Here's how the part is built. I have some questions about the finished solid (model axes, mm). A direction names the side the tool comes from. Round coordinates to 2 decimals unless told otherwise and drop trailing zeros. Write each loop counter-clockwise with the first axis right and the second up, starting at its lowest first coordinate (ties: lowest second). Pieces come first, ordered by that corner, then holes. Notation, with made-up numbers: (24, 25.25) -> (82, 25.25) arc R27 ccw to (82, 48.25) -> close; hole circle Ø2 at (71, 44.5). An arc over 180 degrees is marked (long way). Answer in a Markdown table with one row per item.
from build123d import *

# Parameters (mm, degrees)
SKETCH1_W           = 10
SKETCH1_H           = 14
SKETCH1_R           = 2.1
BOSS_EXTRUDE1_DEPTH = 2
SKETCH2_W           = 1.8
SKETCH2_H           = 13.4
BOSS_EXTRUDE2_DEPTH = 5
SKETCH3_W           = 1.8
SKETCH3_H           = 1.8
CUT_EXTRUDE1_DEPTH  = 9
SKETCH5_W           = 12.2
SKETCH5_H           = 17
BOSS_EXTRUDE4_DEPTH = 2
SKETCH6_W           = 14
SKETCH6_H           = 5
SKETCH6_W_2         = 0.5
CUT_EXTRUDE2_DEPTH  = 14
SKETCH7_W           = 10
SKETCH7_H           = 2
BOSS_EXTRUDE5_DEPTH = 3


with BuildPart() as part:
    # Sketch1 → Boss-Extrude1 (new body)
    with BuildSketch(Plane(origin=(0, 0, 0), x_dir=(1, 0, 0), z_dir=(0, 1, 0))):
        Rectangle(SKETCH1_W, SKETCH1_H)
        Circle(SKETCH1_R, mode=Mode.SUBTRACT)
        Polygon((5, 7), (5, -7), (5, -8.5), (19, -8.5), (19, 8.5), (5, 8.5), align=None)
    extrude(amount=BOSS_EXTRUDE1_DEPTH)

    # Sketch2 → Boss-Extrude2 (add)
    with BuildSketch(Plane(origin=(0, 2, 0), x_dir=(1, 0, 0), z_dir=(0, 1, 0))):
        Polygon((17.2, 6.7), (19, 6.7), (19, 8.5), (5, 8.5), (5, 7), (5, 6.7), align=None)
        with Locations((18.1, 0)):
            Rectangle(SKETCH2_W, SKETCH2_H)
        Polygon((5, -7), (5, -8.5), (19, -8.5), (19, -6.7), (17.2, -6.7), (5, -6.7), align=None)
    extrude(amount=BOSS_EXTRUDE2_DEPTH)

    # Sketch3 → Cut-Extrude1 (cut)
    with BuildSketch(Plane(origin=(0, 7, 0), x_dir=(1, 0, 0), z_dir=(0, 1, 0))):
        Polygon((19, -6.7), (19, 8.5), (17.2, 8.5), (17.2, 6.7), (17.2, -6.7), align=None)
        with Locations((18.1, -7.6)):
            Rectangle(SKETCH3_W, SKETCH3_H)
    extrude(amount=-CUT_EXTRUDE1_DEPTH, mode=Mode.SUBTRACT)

    # Sketch5 → Boss-Extrude4 (add)
    with BuildSketch(Plane(origin=(0, 7, 0), x_dir=(1, 0, 0), z_dir=(0, 1, 0))):
        with Locations((11.1, 0)):
            Rectangle(SKETCH5_W, SKETCH5_H)
    extrude(amount=BOSS_EXTRUDE4_DEPTH)

    # Sketch6 → Cut-Extrude2 (cut)
    with BuildSketch(Plane.ZY.offset(-5)):
        with Locations((0, 4.5)):
            Rectangle(SKETCH6_W, SKETCH6_H)
        with Locations((-7.25, 4.5)):
            Rectangle(SKETCH6_W_2, SKETCH6_H)
        with Locations((7.25, 4.5)):
            Rectangle(SKETCH6_W_2, SKETCH6_H)
    extrude(amount=-CUT_EXTRUDE2_DEPTH, mode=Mode.SUBTRACT)

    # Sketch7 → Boss-Extrude5 (add)
    with BuildSketch(Plane(origin=(0, 0, -7), x_dir=(-1, 0, 0), z_dir=(0, 0, -1))):
        with Locations((0, 1)):
            Rectangle(SKETCH7_W, SKETCH7_H)
    extrude(amount=BOSS_EXTRUDE5_DEPTH)


solid = part.part
1) I want a section at B-B, the plane z = -2.5. List the corners of the cut face in (x, y) for me, and give its area (3 significant figures).
Response:
| item | result |
|---|---|
| outline | (-5, 0) -> (17.2, 0) -> (17.2, 2) -> (-5, 2) -> close; (5, 7) -> (17.2, 7) -> (17.2, 9) -> (5, 9) -> close |
| area | 68.8 mm^2 |
2) I need wall thicknesses on line 1 (X direction, y = 1.3, z = 0); line 2 (Y direction, x = 15.25, z = -2.5); line 3 (Z direction, x = 0, y = 1.2). Which ranges of each line are inside material? Lowest first, please. Write a range as [from, to].
Response:
| item | result |
|---|---|
| line 1 | x = [-5, -2.1], [2.1, 17.2] |
| line 2 | y = [0, 2], [7, 9] |
| line 3 | z = [-10, -2.1], [2.1, 7] |
3) I want a section at A-A, the plane x = 0. List the corners of the cut face in (y, z) for me.
Response:
| item | result |
|---|---|
| outline | (0, -10) -> (2, -10) -> (2, -2.1) -> (0, -2.1) -> close; (0, 2.1) -> (2, 2.1) -> (2, 7) -> (0, 7) -> close |
4) For pin 1 (2.5 mm diameter, centred on x = 13.5, y = 5, fed in from -Z); pin 2 (1.5 mm diameter, centred on x = 0, z = -8, fed in from +Y); pin 3 (4 mm diameter, centred on x = 0, z = 0, fed in from +Y); pin 4 (5 mm diameter, centred on y = 8, z = 2, fed in from -X), each with a flat end and sliding along its axis, tell me the tip position at first contact or that it passes through.
Response:
| item | result |
|---|---|
| pin 1 | stops at z = -8.5 |
| pin 2 | stops at y = 2 |
| pin 3 | passes through |
| pin 4 | stops at x = 5 |
5) Which directions (+Z, -Z, +X, -X, +Y, -Y) give clear straight access to the entire face, cutting with the end or side of a thin tool? Please do faces 4 (the face through (0, 1, 7)), 5 (the face through (11, 4, -8.5)), 6 (the face through (11, 7, 0)).
Response:
| item | result |
|---|---|
| face 4 | +Z, -X, +Y, -Y |
| face 5 | -Z, +X, +Y, -Y |
| face 6 | +X, -X |
6) I want a section at D-D, the plane x = 13.5. List the corners of the cut face in (y, z) for me.
Response:
| item | result |
|---|---|
| outline | (0, -8.5) -> (9, -8.5) -> (9, 8.5) -> (0, 8.5) -> close; hole (2, -7.5) -> (7, -7.5) -> (7, 7.5) -> (2, 7.5) -> close |
7) We'd pull the mould along Y, two halves only. Please class faces 1 (the face through (6, 0, -1)), 2 (the face through (5, 1, -9)), 3 (the face through (11, 4, 7.5)): +Y half, -Y half, draft (parallel to the pull), parting line (faces both ways), or undercut.
Response:
| item | result |
|---|---|
| face 1 | -Y half |
| face 2 | draft |
| face 3 | undercut |
8) I want a section at C-C, the plane z = 0. List the corners of the cut face in (x, y) for me.
Response:
| item | result |
|---|---|
| outline | (-5, 0) -> (-2.1, 0) -> (-2.1, 2) -> (-5, 2) -> close; (2.1, 0) -> (17.2, 0) -> (17.2, 2) -> (2.1, 2) -> close; (5, 7) -> (17.2, 7) -> (17.2, 9) -> (5, 9) -> close |
